Design review of the part built by this model. Coordinates are the model's own, in mm. A direction names the side the tool comes from. Round coordinates to 2 decimals unless told otherwise and drop trailing zeros. Write each loop counter-clockwise with the first axis right and the second up, starting at its lowest first coordinate (ties: lowest second). Pieces come first, ordered by that corner, then holes. Notation, with made-up numbers: (30.25, 33) -> (89.25, 33) arc R21 ccw to (89.25, 67) -> close; hole circle Ø4 at (67, 7). An arc over 180 degrees is marked (long way). Write item = value, one per line. Start each with the question number.
Item 1: Add section D-D, the plane x = 7. State the section outline as (y, z) points, then the cut area to 3 significant figures.
Item 2: Add section A-A, the plane x = 64.25. State the section outline as (y, z) points, then the cut area to 3 significant figures.
Item 3: To check wall thickness, follow L1, parallel to Z at x = 3.25, y = 0.8; L2, parallel to X at y = 0.75, z = -3.25; L3, parallel to X at y = 2, z = -28. State the ranges of each line that lie inside material, in increasing order.
Item 4: Machinability: for faces 5 (the flat face through (67.5, 6, -21)), 6 (the flat face through (4, 8, -16.5)), 7 (the flat face through (11, 8, -27)), 8 (the flat face through (57, 8, -27)), 9 (the flat face through (63, 8, -16.5)), which of the approach directions +Z, -Z, +X, -X, +Y, -Y give a long, thin tool a straight path to every point of the face, cutting with its end or side? Answer none if there is none.
Item 5: Add section C-C, the plane y = 9. State the section outline as (x, z) points, then the cut area to 3 significant figures.
Item 6: For pin 1 Ø5.5 at (x, z) = (64.25, -3.25) entering from +Y; pin 2 Ø6 at (x, z) = (60, -28.5) entering from +Y; pin 3 Ø2 at (y, z) = (12, -30) entering from +X; pin 4 Ø4 at (y, z) = (5.5, -6.5) entering from +X, all flat-tipped, find the tip position at first contact; note any pin that passes through.
Item 7: Add section B-B, the plane z = -40.25. State the section outline as (x, y) points, then the cut area to 3 significant figures.
Item 8: Mouldability with a two-part tool opening along X and no side actions: class faces 1 (the flat face through (22.25, 8, -35)), 2 (the flat face through (33, 7, 0)), 3 (the cylindrical face through (65.919, 0.74, -3.776)), 4 (the cylindrical face through (2.87, 0.74, -1.54)) as released by +X, released by -X, zero draft, split by the parting line, or undercut.
from build123d import *

# Parameters (mm, degrees)
ESQUISSE1_W        = 67.5
ESQUISSE1_H        = 43.5
ESQUISSE1_R        = 1.75
BOSS_EXTRU_1_DEPTH = 1.5
BOSS_EXTRU_2_DEPTH = 13


with BuildPart() as part:
    # Esquisse1 → Boss.-Extru.1 (new body)
    with BuildSketch(Plane(origin=(0, 0, 0), x_dir=(1, 0, 0), z_dir=(0, 1, 0))):
        with Locations((33.75, 21.75)):
            Rectangle(ESQUISSE1_W, ESQUISSE1_H)
        with Locations((3.25, 40.25)):
            Circle(ESQUISSE1_R, mode=Mode.SUBTRACT)
        with Locations((64.25, 40.25)):
            Circle(ESQUISSE1_R, mode=Mode.SUBTRACT)
        with Locations((64.25, 3.25)):
            Circle(ESQUISSE1_R, mode=Mode.SUBTRACT)
        with Locations((3.25, 3.25)):
            Circle(ESQUISSE1_R, mode=Mode.SUBTRACT)
    extrude(amount=BOSS_EXTRU_1_DEPTH)

    # Esquisse3 → Boss.-Extru.2 (add)
    with BuildSketch(Plane(origin=(0, 1.5, 0), x_dir=(1, 0, 0), z_dir=(0, 1, 0))):
        Polygon((45.25, 43.5), (22.25, 43.5), (22.25, 27), (0, 27), (0, 16.5), (8, 16.5), (8, 0), (59.5, 0), (59.5, 16.5), (67.5, 16.5), (67.5, 27), (45.25, 27), align=None)
    extrude(amount=BOSS_EXTRU_2_DEPTH)


solid = part.part
Result set:
q1.outline = (0, -43.5) -> (1.5, -43.5) -> (1.5, -27) -> (14.5, -27) -> (14.5, -16.5) -> (1.5, -16.5) -> (1.5, 0) -> (0, 0) -> close
q1.area = 202 mm²
q2.outline = (0, -43.5) -> (1.5, -43.5) -> (1.5, -42) -> (0, -42) -> close; (0, -38.5) -> (1.5, -38.5) -> (1.5, -27) -> (14.5, -27) -> (14.5, -16.5) -> (1.5, -16.5) -> (1.5, -5) -> (0, -5) -> close; (0, -1.5) -> (1.5, -1.5) -> (1.5, 0) -> (0, 0) -> close
q2.area = 191 mm²
q3.L1 = -43.5 to -42, -38.5 to -5, -1.5 to 0
q3.L2 = 0 to 1.5, 5 to 62.5, 66 to 67.5
q3.L3 = 22.25 to 45.25
q4.face_5 = +Z, -Z, +X, +Y, -Y
q4.face_6 = +Z, -X, +Y
q4.face_7 = -Z, -X, +Y
q4.face_8 = -Z, +X, +Y
q4.face_9 = +Z, +X, +Y
q5.outline = (0, -27) -> (22.25, -27) -> (22.25, -43.5) -> (45.25, -43.5) -> (45.25, -27) -> (67.5, -27) -> (67.5, -16.5) -> (59.5, -16.5) -> (59.5, 0) -> (8, 0) -> (8, -16.5) -> (0, -16.5) -> close
q5.area = 1,940 mm²
q6.pin_1 = 1.5
q6.pin_2 = 14.5
q6.pin_3 = 45.25
q6.pin_4 = 59.5
q7.outline = (0, 0) -> (1.5, 0) -> (1.5, 1.5) -> (0, 1.5) -> close; (5, 0) -> (62.5, 0) -> (62.5, 1.5) -> (45.25, 1.5) -> (45.25, 14.5) -> (22.25, 14.5) -> (22.25, 1.5) -> (5, 1.5) -> close; (66, 0) -> (67.5, 0) -> (67.5, 1.5) -> (66, 1.5) -> close
q7.area = 390 mm²
q8.face_1 = released by -X
q8.face_2 = zero draft
q8.face_3 = undercut
q8.face_4 = undercut
